For this review, take the finished solid that the model builds, in its own axes (mm). Face numbers are marked on the shaded views. Round coordinates to 2 decimals unless told otherwise and drop trailing zeros. Write each loop counter-clockwise with the first axis right and the second up, starting at its lowest first coordinate (ties: lowest second). Pieces come first, ordered by that corner, then holes. Notation, with made-up numbers: (24.25, 13.5) -> (71.25, 13.5) arc R28 ccw to (71.25, 38.5) -> close; hole circle Ø5 at (57.5, -37). An arc over 180 degrees is marked (long way). Answer in a Markdown table with one row per item.
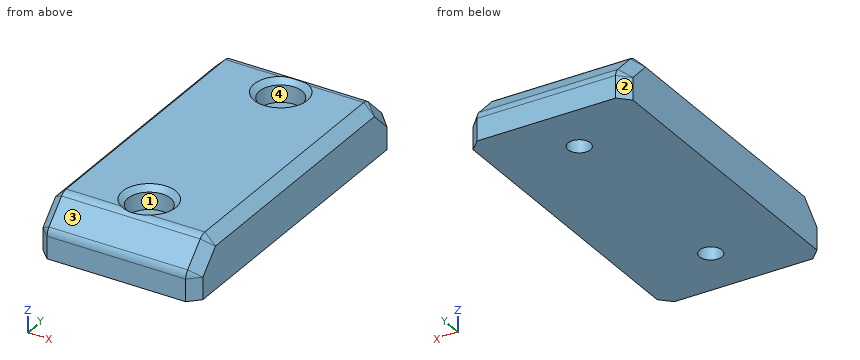
Autodesk Inventor part; units mm, degrees
ref_plane "YZ Plane" through (0, 0, 0) normal (1, 0, 0) x (0, 1, 0)
ref_plane "XZ Plane" through (0, 0, 0) normal (0, 1, 0) x (-1, 0, 0)
ref_plane "XY Plane" through (0, 0, 0) normal (0, 0, 1) x (1, 0, 0)
sketch "スケッチ1" plane through (0, 0, 0) normal (0, 0, 1) x (1, 0, 0)
  line L0 (-15, -30) -> (15, -30)
  line L1 (15, -30) -> (15, 30)
  line L2 (15, 30) -> (-15, 30)
  line L3 (-15, 30) -> (-15, -30)
  line L4 (-15, -30) -> (15, 30) construction
  line L5 (15, -30) -> (-15, 30) construction
  point P0 (0, 0)
  dimension "d0" = 30
  dimension "d1" = 60
extrude "押し出し1" add sketch "スケッチ1" along normal blind 10
chamfer "面取り1" distance 5 angle 45 2 edges at (0, 30, 10) (0, -30, 10)
fillet "フィレット1" radius 2 4 edges at (0, 30, 5) (0, 25, 10) (0, -25, 10) (0, -30, 5)
chamfer "面取り2" distance 2 angle 45 18 edges at (15, 0, 10) (15, 24.9369, 9.8478) (15, 27.5, 7.5) (15, 29.8478, 4.9369) (15, 30, 2.0858) (15, -24.9369, 9.8478) (15, -27.5, 7.5) (15, -29.8478, 4.9369) (15, -30, 2.0858) (-15, 0, 10) (-15, -24.9369, 9.8478) (-15, -27.5, 7.5) (-15, -29.8478, 4.9369) (-15, -30, 2.0858) (-15, 24.9369, 9.8478) (-15, 27.5, 7.5) (-15, 29.8478, 4.9369) (-15, 30, 2.0858)
sketch "スケッチ2" plane through (0, 0, 10) normal (0, 0, 1) x (1, 0, 0)
  line L0 (-13, -24.1716) -> (-13, 24.1716)
  line L1 (13, -24.1716) -> (-13, -24.1716)
  line L2 (13, 24.1716) -> (13, -24.1716)
  line L3 (-13, 24.1716) -> (13, 24.1716)
  point P0 (0, 0)
  point P1 (0, 20)
  point P2 (0, -20)
  dimension "d11" = 40
  dimension "d12" = 20
hole "穴1" at (0, 20, 10) at (0, -20, 10) direction (0, 0, -1) diameter 4.2 depth 21.5 counterbore diameter 8 counterbore depth 4.2
chamfer "面取り3" distance 1 angle 45 2 edges at (0, 24, 10) (0, -16, 10)
properties part number "Flame_Cover"
1) Consider section D-D on x = 0. State the section outline as (y, z) points.
Solved:
| item | result |
|---|---|
| outline | (-30, 0) -> (-22.1, 0) -> (-22.1, 5.8) -> (-24, 5.8) -> (-24, 9) -> (-24.87, 9.87) arc R2 ccw to (-25.59, 9.41) -> (-29.41, 5.59) arc R2 ccw to (-30, 4.17) -> close; (-17.9, 0) -> (17.9, 0) -> (17.9, 5.8) -> (16, 5.8) -> (16, 9) -> (15, 10) -> (-15, 10) -> (-16, 9) -> (-16, 5.8) -> (-17.9, 5.8) -> close; (22.1, 0) -> (30, 0) -> (30, 4.17) arc R2 ccw to (29.41, 5.59) -> (25.59, 9.41) arc R2 ccw to (24.87, 9.87) -> (24, 9) -> (24, 5.8) -> (22.1, 5.8) -> close |
2) Consider section B-B on y = -20. State the section outline as (x, z) points, then the cut area to 3 significant figures.
Solved:
| item | result |
|---|---|
| outline | (-15, 0) -> (-2.1, 0) -> (-2.1, 5.8) -> (-4, 5.8) -> (-4, 9) -> (-5, 10) -> (-13, 10) -> (-15, 8) -> close; (2.1, 0) -> (15, 0) -> (15, 8) -> (13, 10) -> (5, 10) -> (4, 9) -> (4, 5.8) -> (2.1, 5.8) -> close |
| area | 237 mm² |
3) Clearance check with flat-ended pins moving along their axes: pin 1 Ø4 at (x, y) = (6.5, 16) entering from -Z; pin 2 Ø4 at (x, y) = (-1, -22) entering from +Z; pin 3 Ø9 at (x, y) = (0, -20) entering from +Z. State where each tip first meets the part, or that it passes through.
Solved:
| item | result |
|---|---|
| pin 1 | z = 0 |
| pin 2 | z = 9.24 |
| pin 3 | z = 9.5 |
4) Consider section C-C on x = 7.5. State the section outline as (y, z) points.
Solved:
| item | result |
|---|---|
| outline | (-30, 0) -> (30, 0) -> (30, 4.17) arc R2 ccw to (29.41, 5.59) -> (25.59, 9.41) arc R2 ccw to (24.17, 10) -> (-24.17, 10) arc R2 ccw to (-25.59, 9.41) -> (-29.41, 5.59) arc R2 ccw to (-30, 4.17) -> close |
5) For line 1 (Y direction, x = 0, z = 1.8); line 2 (X direction, y = 20, z = 7.15); line 3 (Y direction, x = 0, z = 6.5), list the stretches that pass through material, from the lowest coordinate up. Write a range as [from, to].
Solved:
| item | result |
|---|---|
| line 1 | [-30, -22.1], [-17.9, 17.9], [22.1, 30] |
| line 2 | [-15, -4], [4, 15] |
| line 3 | [-28.5, -24], [-16, 16], [24, 28.5] |
6) Mouldability with a two-part tool opening along Y and no side actions: class the marked faces 1, 2, 3 and 4 as pulls with the +Y half, pulls with the -Y half, needs draft (parallel to the pull), parting line crosses it, or undercut.
Solved:
| item | result |
|---|---|
| face 1 | undercut |
| face 2 | pulls with the +Y half |
| face 3 | pulls with the -Y half |
| face 4 | undercut |
7) Consider section A-A on z = 2.25. State the section outline as (x, y) points.
Solved:
| item | result |
|---|---|
| outline | (-15, -28) -> (-13, -30) -> (13, -30) -> (15, -28) -> (15, 28) -> (13, 30) -> (-13, 30) -> (-15, 28) -> close; hole circle Ø4.2 at (0, -20); hole circle Ø4.2 at (0, 20) |
